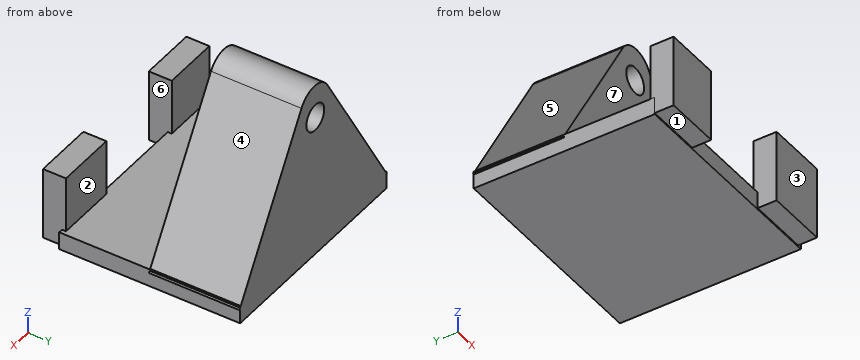
```python
from build123d import *

# Parameters (mm, degrees)
F0_R     = 3.753216
F1_DEPTH = 25.4
F3_DEPTH = 50.8
F4_W     = 15.826155
F4_H     = 6.447691
F4_W_2   = 16.998462
F5_DEPTH = 20.32


with BuildPart() as f1:
    # F0 (on Front) → F1 (new body)
    with BuildSketch(Plane.XZ):
        with BuildLine():
            Line((-8.156309, 26.172908), (-33.264231, -16.558846))
            Line((-33.264231, -16.558846), (28.868075, -16.558846))
            Line((28.868075, -16.558846), (2.739173, 26.263524))
            ThreePointArc((2.739173, 26.263524), (-2.734247, 29.305814), (-8.156309, 26.172908))
        make_face()
        with Locations((-3.077308, 19.782692)):
            Circle(F0_R, mode=Mode.SUBTRACT)
    extrude(amount=F1_DEPTH)

    # F2 (on Front) → F3 (join)
    with BuildSketch(Plane.XZ):
        Polygon((28.574998, -15.679616), (-32.971155, -15.679616), (-32.971155, -20.661924), (-18.911924, -20.661924), (11.673916, -20.661924), (28.574998, -20.661924), align=None)
    extrude(amount=F3_DEPTH)

    # F4 (on Top) → F5 (join)
    with BuildSketch(Plane.XY):
        with Locations((-25.058077, -52.900384)):
            Rectangle(F4_W, F4_H)
        with Locations((18.903461, -52.900384)):
            Rectangle(F4_W_2, F4_H)
    extrude(amount=-F5_DEPTH)


solid = f1.part
```
CAD build for the part. Positions are in the model's coordinates, mm. Face numbers are marked on the shaded views. A direction names the side the tool comes from. Coordinates: 2 decimals unless noted, no trailing zeros. Loops run counter-clockwise (first coordinate to the right, second up) from the corner with the lowest first, then second, coordinate; pieces in that order, holes last. Notation, with made-up numbers: (31, 18) - (59, 18) arc R11 cw to (59, 25) - close; hole circle Ø5 at (41.25, 59.25). An arc over 180 degrees is marked (long way). Use CSV: the item, a comma, the result in double quotes. Start each with the question number.
Q1. Probe probe 1 along Y at (x, z) = (16.5, -8); probe 2 along Z at (x, y) = (-19, -39.5); probe 3 along Y at (x, z) = (10, -9). List the from-to ranges inside material, lowest first. Write a range as from..to.
Q2. Cut at C-C, the plane x = -23. List the corners of the cut face in (y, z), then the cut area to 3 significant figures.
Q3. Drop flat-ended pins along their axis: P1, Ø2, axis at x = -0.5, y = -31, coming from the +Z side; P2, Ø4.5, axis at x = -23.5, z = -11, coming from the +Y side; P3, Ø22.5, axis at x = -5, z = -2, coming from the -Y side; P4, Ø3, axis at x = -29, y = -52.5, coming from the +Z side. Give the stop position or say it passes through.
Q4. 3-axis set-ups, long thin cutter, end or side, ignore diameter. For the marked faces 4, 5, 6 and 7: which of +Z, -Z, +X, -X, +Y, -Y reach the whole face in a straight line?
Q5. Two-plate mould, pull along Y, no slides. Class the marked faces 1, 2 and 3: +Y half, -Y half, draft (parallel to the pull), parting line (faces both ways), or undercut.
Q6. Cut at D-D, the plane y = -11. List the corners of the cut face in (x, z) (3 decimals), then the cut area to 3 significant figures.
Q7. Cut at B-B, the plane z = -6.5. List the corners of the cut face in (x, y) (3 decimals), then the cut area to 3 significant figures.
Q8. Cut at A-A, the plane x = -5.5. List the corners of the cut face in (y, z).
Here are the results:
1,probe 1,"-56.12..-49.68, -25.4..0"
1,probe 2,"-20.66..-15.68"
1,probe 3,"-25.4..0"
2,outline,"(-56.12, -20.32) - (-50.8, -20.32) - (-50.8, -20.66) - (0, -20.66) - (0, 0.91) - (-25.4, 0.91) - (-25.4, -15.68) - (-49.68, -15.68) - (-49.68, 0) - (-56.12, 0) - close"
2,area,"800 mm2"
3,P1,"z = -15.68"
3,P2,"y = 0"
3,P3,"y = -25.4"
3,P4,"z = 0"
4,face 4,"+Z, +X, +Y"
4,face 5,"+Z, -X, +Y"
4,face 6,"+Z, -Y"
4,face 7,"+Z, +X, -X"
5,face 1,"draft"
5,face 2,"undercut"
5,face 3,"-Y half"
6,outline,"(-33.264, -16.559) - (-32.971, -16.559) - (-32.971, -20.662) - (28.575, -20.662) - (28.575, -16.559) - (28.868, -16.559) - (28.575, -16.079) - (28.575, -15.68) - (28.332, -15.68) - (2.739, 26.264) arc R6.35 ccw to (-8.156, 26.173) - (-32.748, -15.68) - (-32.971, -15.68) - (-32.971, -16.06) - close; hole circle Ø7.506 at (-3.077, 19.783)"
6,area,"1,790 mm2"
7,outline,"(-32.971, -56.124) - (-17.145, -56.124) - (-17.145, -49.677) - (-32.971, -49.677) - close; (-27.354, -25.4) - (22.73, -25.4) - (22.73, 0) - (-27.354, 0) - close; (10.404, -56.124) - (27.403, -56.124) - (27.403, -49.677) - (10.404, -49.677) - close"
7,area,"1,480 mm2"
8,outline,"(-50.8, -20.66) - (0, -20.66) - (0, 16.92) - (-25.4, 16.92) - (-25.4, -15.68) - (-50.8, -15.68) - close; (-25.4, 22.65) - (0, 22.65) - (0, 28.65) - (-25.4, 28.65) - close"
